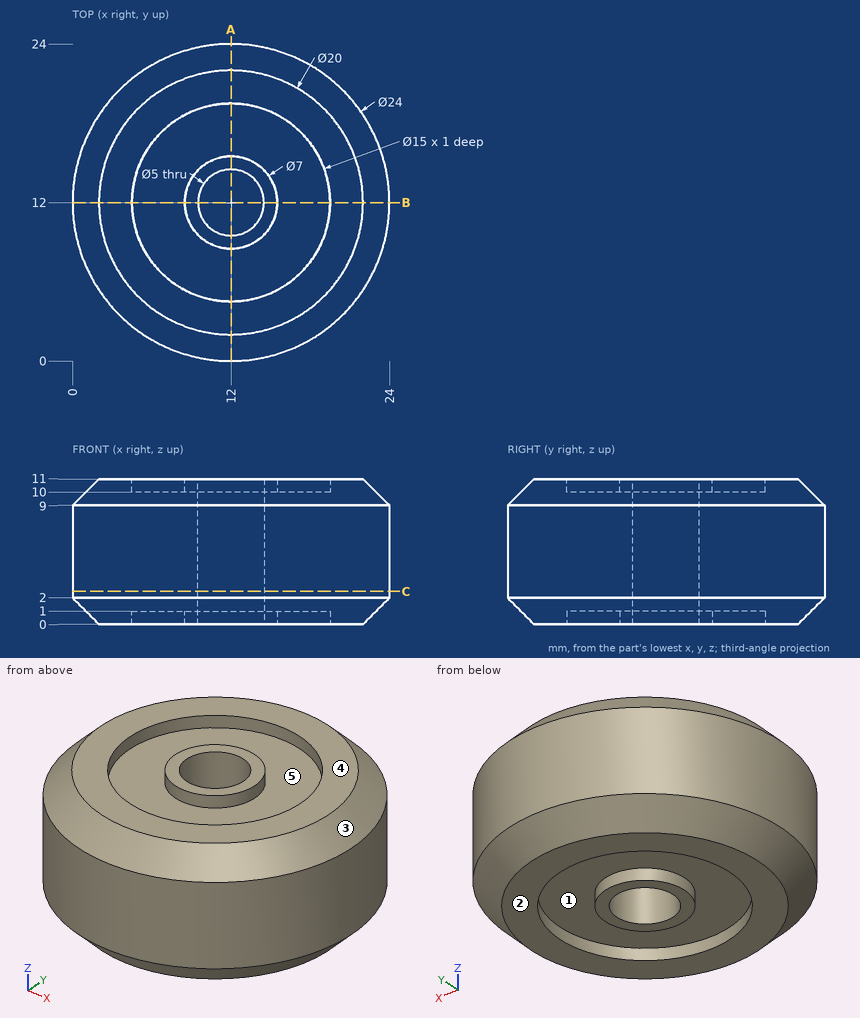
Geometry check sheet. Reference: drawing and pictorial views, mm from the part's lowest x, y, z. A direction names the side the tool comes from. Coordinates: 2 decimals unless noted, no trailing zeros. Order: outer loops, then holes, each group sorted by start corner. A loop starts at its lowest first (then second) coordinate and runs counter-clockwise, first axis right, second up. Notation, with made-up numbers: (54, -18) - (88, -18) arc R4 cw to (88, -14) - close; hole circle Ø7 at (-6.75, 9). An arc over 180 degrees is marked (long way). Answer in a Markdown table with one row per item. Add a question column.
1) Material ranges on line 1 along Y through (x, z) = (11, 10.25); line 2 along Y through (x, z) = (12, 0.4); line 3 along X through (y, z) = (12.5, 2.5), recorded low to high. Write a range as [from, to].
2) Set-up check for the marked faces 1 and 2: record each of +Z, -Z, +X, -X, +Y, -Y from which the full face is reachable in a straight line by a thin tool's end or side.
3) Cross-section at C-C, the plane z = 2.5. Record the cut outline in (x, y), then the cut area to 3 significant figures.
4) Gauge pin test, flat ends, axial feed: P1, Ø1, axis at x = 9, z = 2.5, coming from the +Y side; P2, Ø1, axis at y = 6, z = 8, coming from the -X side; P3, Ø1.5, axis at y = 20.5, z = 2.5, coming from the +X side. Record the tip position at first contact, or that the pin passes through.
5) Cross-section at A-A, the plane x = 12. Record the cut outline in (y, z).
6) Release check for a two-part mould opening along X. For the marked faces 3, 4 and 5 record: +X half, -X half, draft (parallel to the pull), parting line (faces both ways), or undercut.
Check result:
| question | item | result |
|---|---|---|
| 1 | line 1 | y = [1.3, 4.57], [8.65, 9.71], [14.29, 15.35], [19.43, 22.7] |
| 1 | line 2 | y = [1.6, 4.5], [8.5, 9.5], [14.5, 15.5], [19.5, 22.4] |
| 1 | line 3 | x = [0.01, 9.55], [14.45, 23.99] |
| 2 | face 1 | -Z |
| 2 | face 2 | -Z, +X, -X, +Y, -Y |
| 3 | outline | circle Ø24 at (12, 12); hole circle Ø5 at (12, 12) |
| 3 | area | 433 mm² |
| 4 | P1 | stops at y = 23.74 |
| 4 | P2 | stops at x = 1.33 |
| 4 | P3 | stops at x = 21.16 |
| 5 | outline | (0, 2) - (2, 0) - (4.5, 0) - (4.5, 1) - (8.5, 1) - (8.5, 0) - (9.5, 0) - (9.5, 11) - (8.5, 11) - (8.5, 10) - (4.5, 10) - (4.5, 11) - (2, 11) - (0, 9) - close; (14.5, 0) - (15.5, 0) - (15.5, 1) - (19.5, 1) - (19.5, 0) - (22, 0) - (24, 2) - (24, 9) - (22, 11) - (19.5, 11) - (19.5, 10) - (15.5, 10) - (15.5, 11) - (14.5, 11) - close |
| 6 | face 3 | parting line |
| 6 | face 4 | draft |
| 6 | face 5 | undercut |
